from build123d import *

# Parameters (mm, degrees)
F1_DEPTH  = 10
F2_W      = 15
F2_H      = 42.8
F3_DEPTH  = 3
F4_R      = 1.35
F5_DEPTH  = 7.001
F6_W      = 4
F6_H      = 4.6
F6_H_2    = 42.8
F7_DEPTH  = 8
F8_DEPTH  = 10
F9_R      = 2.2
F10_DEPTH = 4.001


with BuildPart() as f1:
    # F0 (on Right) → F1 (new body)
    with BuildSketch(Plane.YZ):
        Polygon((7, 0), (-23, 0), (-23, -42.8), (0, -42.8), (7, -42.8), align=None)
    extrude(amount=F1_DEPTH)

    # F2 (on face) → F3 (cut)
    with BuildSketch(Plane.YZ.offset(10)):
        with Locations((-15.5, -21.4)):
            Rectangle(F2_W, F2_H)
    extrude(amount=-F3_DEPTH, mode=Mode.SUBTRACT)

    # F4 (on face) → F5 (cut, through all)
    with BuildSketch(Plane.YZ.offset(7)):
        with Locations((-15.5, -21.4)):
            Circle(F4_R)
        with Locations((-15.5, -11.4)):
            Circle(F4_R)
        with Locations((-15.5, -31.4)):
            Circle(F4_R)
    extrude(amount=-F5_DEPTH, mode=Mode.SUBTRACT)

    # F6 (on face) → F7 (join)
    with BuildSketch(Plane(origin=(0, 0, 0), x_dir=(0, -1, 0), z_dir=(-1, 0, 0))):
        with Locations((-5, 2.3)):
            Rectangle(F6_W, F6_H)
        with Locations((-5, -45.1)):
            Rectangle(F6_W, F6_H)
        with Locations((-5, -21.4)):
            Rectangle(F6_W, F6_H_2)
    extrude(amount=F7_DEPTH)

    # F8 (add): faces of the model
    f8_faces = [f1.faces().sort_by_distance(p)[0] for p in [
        (0, 5, -45.1),
        (0, 5, 2.3),
    ]]
    extrude(f8_faces, amount=F8_DEPTH)

    # F9 (on face) → F10 (cut, through all)
    with BuildSketch(Plane.XZ.offset(-3)):
        with Locations((-4, 0.85)):
            Circle(F9_R)
        with Locations((-4, -43.65)):
            Circle(F9_R)
    extrude(amount=-F10_DEPTH, mode=Mode.SUBTRACT)


solid = f1.part
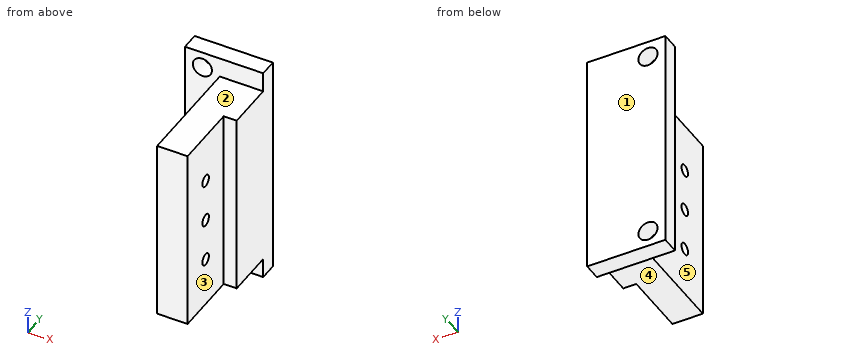
Build history of the part. All positions in model axes, mm. Face numbers are marked on the shaded views. A direction names the side the tool comes from. Coordinates: 2 decimals unless noted, no trailing zeros. Order: outer loops, then holes, each group sorted by start corner. A loop starts at its lowest first (then second) coordinate and runs counter-clockwise, first axis right, second up. Notation, with made-up numbers: (28, 15) - (72, 15) arc R16 ccw to (72, 38) - close; hole circle Ø7 at (13.5, 41.5). An arc over 180 degrees is marked (long way). Write item = value, one per line. Start each with the question number.
1) Wall check: line 1 along Z through (x, y) = (-4, 5.55); line 2 along Z through (x, y) = (3.25, -15.5); line 3 along X through (y, z) = (-7.75, -39.5). Give the ranges that are in metal, low to high. Write a range as from..to.
2) Saw through at A-A on y = -15.5. Write the cut outline in (x, z), then the cut area to 3 significant figures.
3) 3-axis set-ups, long thin cutter, end or side, ignore diameter. For the marked faces 1, 2, 3, 4 and 5: which of +Z, -Z, +X, -X, +Y, -Y reach the whole face in a straight line?
4) Flat gauge pins, fed straight in: pin 1 Ø10 at (x, y) = (3, -18) entering from -Z; pin 2 Ø4 at (y, z) = (-16, -17.5) entering from -X; pin 3 Ø5 at (x, y) = (5.5, -10) entering from +Z. Where does each tip first touch, or does it go through?
5) Saw through at C-C on x = -4. Write the cut outline in (y, z), then the cut area to 3 significant figures.
6) Saw through at B-B on z = -21.4. Write the cut outline in (x, y), then the cut area to 3 significant figures.
7) Saw through at D-D on x = 2.75. Write the cut outline in (y, z).
From the geometry:
q1.line_1 = -47.4..-45.85, -41.45..-1.35, 3.05..4.6
q1.line_2 = -42.8..-32.75, -30.05..-22.75, -20.05..-12.75, -10.05..0
q1.line_3 = 0..10
q2.outline = (0, -42.8) - (7, -42.8) - (7, -32.75) - (0, -32.75) - close; (0, -30.05) - (7, -30.05) - (7, -22.75) - (0, -22.75) - close; (0, -20.05) - (7, -20.05) - (7, -12.75) - (0, -12.75) - close; (0, -10.05) - (7, -10.05) - (7, 0) - (0, 0) - close
q2.area = 243 mm^2
q3.face_1 = +Z, -Z, +X, -X, +Y
q3.face_2 = +Z, +X, -X, -Y
q3.face_3 = +Z, -Z, +X, -Y
q3.face_4 = -Z, +X, -X, -Y
q3.face_5 = +Z, -Z, -X, -Y
q4.pin_1 = -42.8
q4.pin_2 = 0
q4.pin_3 = 0
q5.outline = (3, -47.4) - (7, -47.4) - (7, -45.85) - (3, -45.85) - close; (3, -41.45) - (7, -41.45) - (7, -1.35) - (3, -1.35) - close; (3, 3.05) - (7, 3.05) - (7, 4.6) - (3, 4.6) - close
q5.area = 173 mm^2
q6.outline = (-8, 3) - (0, 3) - (0, -14.15) - (7, -14.15) - (7, -8) - (10, -8) - (10, 7) - (-8, 7) - close; (0, -23) - (7, -23) - (7, -16.85) - (0, -16.85) - close
q6.area = 268 mm^2
q7.outline = (-23, -42.8) - (3, -42.8) - (3, -47.4) - (7, -47.4) - (7, 4.6) - (3, 4.6) - (3, 0) - (-23, 0) - close; hole circle Ø2.7 at (-15.5, -31.4); hole circle Ø2.7 at (-15.5, -21.4); hole circle Ø2.7 at (-15.5, -11.4)
